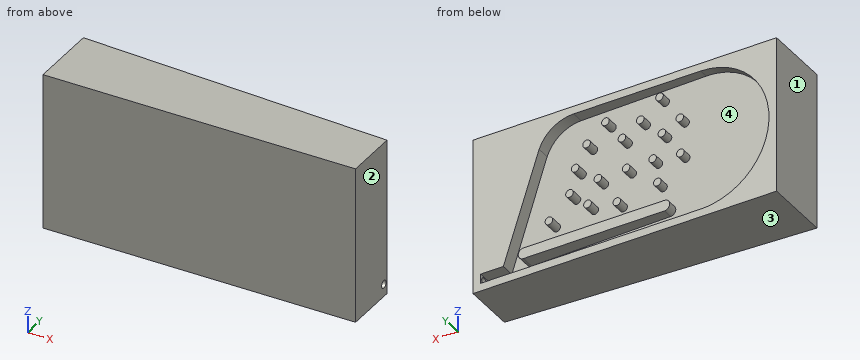
from build123d import *

# Parameters (mm, degrees)
EXTRUDE_1_DEPTH      = 20
CUT_EXTRUDE_START    = 20
SKETCH_4_R           = 0.5
CUT_EXTRUDE_6_DEPTH  = 15
EXTRUDE_2_DEPTH      = 10
EXTRUDE_3_DEPTH      = 20
CUT_EXTRUDE_7_DEPTH  = 20
SKETCH_12_R          = 0.5
CUT_EXTRUDE_10_DEPTH = 20
CUT_EXTRUDE_15_DEPTH = 20
SKETCH_15_R          = 0.5
CUT_EXTRUDE_16_DEPTH = 1


with BuildPart() as part:
    # Sketch 2 → Extrude 1 (new body)
    with BuildSketch(Plane.XY):
        Polygon((0, 0), (0, 20), (40, 15), (40, 0), align=None)
    extrude(amount=EXTRUDE_1_DEPTH)

    # Sketch 4 → Cut-Extrude 6 (cut)
    with BuildSketch(Plane(origin=(1.235539726, 0, 0), x_dir=(1, 0, 0), z_dir=(0, 1, 0)).offset(CUT_EXTRUDE_START)):
        with BuildLine():
            Line((8.764460274, -1), (37.764460274, -1))
            Line((37.764460274, -1), (37.764460274, -19))
            Line((37.764460274, -19), (8.764460274, -19))
            ThreePointArc((8.764460274, -19), (-0.235539726, -10), (8.764460274, -1))
        make_face()
        with Locations(Location((14.484350187, -6.426353647, 0), (0, 0, 180))):
            Circle(SKETCH_4_R, mode=Mode.SUBTRACT)
        with Locations(Location((13.880099762, -12.615834701, 0), (0, 0, 180))):
            Circle(SKETCH_4_R, mode=Mode.SUBTRACT)
        with Locations(Location((18.597641111, -9.629824046, 0), (0, 0, 180))):
            Circle(SKETCH_4_R, mode=Mode.SUBTRACT)
        with Locations(Location((23.67865621, -6.642424392, 0), (0, 0, 180))):
            Circle(SKETCH_4_R, mode=Mode.SUBTRACT)
        with Locations(Location((23.798217352, -14.512669522, 0), (0, 0, 180))):
            Circle(SKETCH_4_R, mode=Mode.SUBTRACT)
        with Locations(Location((19.146558444, -13.71910453, 0), (0, 0, 180))):
            Circle(SKETCH_4_R, mode=Mode.SUBTRACT)
        with Locations(Location((22.321317197, -9.525445181, 0), (0, 0, 180))):
            Circle(SKETCH_4_R, mode=Mode.SUBTRACT)
        with Locations(Location((26.052750908, -8.803862679, 0), (0, 0, 180))):
            Circle(SKETCH_4_R, mode=Mode.SUBTRACT)
        with Locations(Location((25.314084108, -11.850948182, 0), (0, 0, 180))):
            Circle(SKETCH_4_R, mode=Mode.SUBTRACT)
        with Locations(Location((28.771173887, -6.151414905, 0), (0, 0, 180))):
            Circle(SKETCH_4_R, mode=Mode.SUBTRACT)
        with Locations(Location((19.819687009, -5.651663075, 0), (0, 0, 180))):
            Circle(SKETCH_4_R, mode=Mode.SUBTRACT)
        with Locations(Location((11.444186287, -9.199481051, 0), (0, 0, 180))):
            Circle(SKETCH_4_R, mode=Mode.SUBTRACT)
        with Locations(Location((11.529073964, -13.817559785, 0), (0, 0, 180))):
            Circle(SKETCH_4_R, mode=Mode.SUBTRACT)
        with Locations(Location((14.193117081, -17.441077825, 0), (0, 0, 180))):
            Circle(SKETCH_4_R, mode=Mode.SUBTRACT)
        with Locations(Location((16.733650127, -15.295531213, 0), (0, 0, 180))):
            Circle(SKETCH_4_R, mode=Mode.SUBTRACT)
        with Locations(Location((21.311821949, -16.574794778, 0), (0, 0, 180))):
            Circle(SKETCH_4_R, mode=Mode.SUBTRACT)
        with Locations(Location((15.10499253, -9.689628951, 0), (0, 0, 180))):
            Circle(SKETCH_4_R, mode=Mode.SUBTRACT)
        with BuildLine():
            Line((13.53826807, -2.349817412), (32.116451532, -2.349817412))
            ThreePointArc((32.116451532, -2.349817412), (32.806890875, -3.040256756), (32.116451532, -3.730696099))
            Line((32.116451532, -3.730696099), (13.53826807, -3.730696099))
            ThreePointArc((13.53826807, -3.730696099), (12.847828727, -3.040256756), (13.53826807, -2.349817412))
        make_face(mode=Mode.SUBTRACT)
    extrude(amount=-CUT_EXTRUDE_6_DEPTH, mode=Mode.SUBTRACT)

    # Sketch 4_5 → Extrude 2 (add)
    with BuildSketch(Plane(origin=(1.235539726, 0, 0), x_dir=(1, 0, 0), z_dir=(0, 1, 0))):
        with BuildLine():
            Line((37.764460274, -19), (37.764460274, -2.2))
            Line((37.764460274, -2.2), (34.764460274, -2.2))
            Line((34.764460274, -2.2), (30.053349233, -15.898079159))
            ThreePointArc((30.053349233, -15.898079159), (28.25547142, -18.150801067), (25.501205312, -19))
            Line((25.501205312, -19), (37.764460274, -19))
        make_face()
    extrude(amount=EXTRUDE_2_DEPTH)

    # Sketch 9 → Extrude 3 (add)
    with BuildSketch(Plane.XY.offset(20)):
        Polygon((0, 0), (40, 0), (40, 5), (0, 8), align=None)
    extrude(amount=-EXTRUDE_3_DEPTH)

    # Sketch 11 → Cut-Extrude 7 (cut)
    with BuildSketch(Plane.XY.offset(20)):
        Polygon((0, 10), (0, 20), (40, 15), (40, 10), align=None)
    extrude(amount=-CUT_EXTRUDE_7_DEPTH, mode=Mode.SUBTRACT)

    # Sketch 12 → Cut-Extrude 10 (cut)
    with BuildSketch(Plane(origin=(40, 0, 0), x_dir=(0, 0, -1), z_dir=(1, 0, 0))):
        with Locations(Location((-1.6, 9, 0), (0, 0, 90))):
            Circle(SKETCH_12_R)
    extrude(amount=-CUT_EXTRUDE_10_DEPTH, mode=Mode.SUBTRACT)

    # Sketch 14 → Cut-Extrude 15 (cut)
    with BuildSketch(Plane.XY.offset(20)):
        Polygon((40, 10), (0, 10), (0, 9), (40, 7), align=None)
    extrude(amount=-CUT_EXTRUDE_15_DEPTH, mode=Mode.SUBTRACT)

    # Sketch 15 → Cut-Extrude 16 (cut)
    with BuildSketch(Plane(origin=(40, 0, 0), x_dir=(0, 0, -1), z_dir=(1, 0, 0))):
        with Locations(Location((-1.6, 6.3, 0), (0, 0, 90))):
            Circle(SKETCH_15_R)
    extrude(amount=-CUT_EXTRUDE_16_DEPTH, mode=Mode.SUBTRACT)


solid = part.part
Build history of the part. All positions in model axes, mm. Face numbers are marked on the shaded views. Give positions to 0.01 mm unless a question says otherwise; leave off trailing zeros. Order: outer loops, then holes, each group sorted by start corner. A loop starts at its lowest first (then second) coordinate and runs counter-clockwise, first axis right, second up. Notation, with made-up numbers: M 51.5,-18.5 L 83.5,-18.5 A17 ccw 83.5,-10.5 Z; hole C 68,-12.5 d10. An arc over 180 degrees is marked long. Use one line per item in the form item = value.
1) Saw through at C-C (x = 5). Give the cut face in (y, z) (3 decimals).
Calculated:
outline = M 0,0 L 8.75,0 L 8.75,2.517 L 7.625,2.517 L 7.625,17.483 L 8.75,17.483 L 8.75,20 L 0,20 Z
2) Saw through at A-A (x = 35.5). Give the cut face in (y, z) (1 decimal), plus the area to 3 significant figures.
Calculated:
outline = M 0,0 L 7.2,0 L 7.2,1 L 5.3,1 L 5.3,3.7 L 7.2,3.7 L 7.2,20 L 0,20 Z
area = 139 mm2
3) Two-plate mould, pull along X, no slides. Class the marked faces 1, 2, 3 and 4: released by +X, released by -X, zero draft, split by the parting line, or undercut.
Calculated:
face_1 = released by -X
face_2 = released by +X
face_3 = zero draft
face_4 = undercut
4) Saw through at B-B (z = 1.6). Give the cut face in (x, y) (3 decimals), plus the area to 3 significant figures.
Calculated:
outline = M 0,0 L 40,0 L 40,5.8 L 39,5.8 L 39,5.075 L 6.769,7.492 L 6.769,8.662 L 0,9 Z; M 39,6.8 L 40,6.8 L 40,7 L 39,7.05 Z
area = 268 mm2
5) Drop a flat-ended pin along its axis: pin 1 (3 mm diameter, centred on x = 19, y = 7.5, fed in from -Z). Give the stop position or say it passes through.
Calculated:
pin_1 = 0
6) Probe probe 1 along Z at (x, y) = (39.8, 6.3); probe 2 along Z at (x, y) = (30, 6); probe 3 along Y at (x, z) = (23, 17) (3 decimals). List the from-to ranges inside material, lowest first.
Calculated:
probe_1 = 0 to 1.1, 2.1 to 20
probe_2 = 0 to 1, 2.35 to 3.73, 5.65 to 6.65, 17.75 to 20
probe_3 = 0 to 6.275
7) Saw through at D-D (x = 29). Give the cut face in (y, z) (3 decimals), plus the area to 3 significant figures.
Calculated:
outline = M 0,0 L 7.55,0 L 7.55,1 L 5.825,1 L 5.825,2.35 L 7.55,2.35 L 7.55,3.731 L 5.825,3.731 L 5.825,18.445 L 7.55,18.445 L 7.55,20 L 0,20 Z
area = 123 mm2
